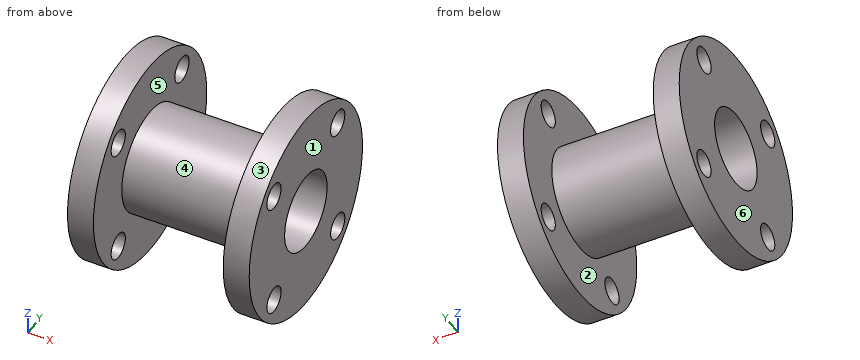
from build123d import *

# Parameters (mm, degrees)
F0_R     = 50.8
F0_R_2   = 6.35
F0_R_3   = 25.4
F1_DEPTH = 12.7
F0_R_4   = 19.05
F2_DEPTH = 88.9
F3_R     = 50.8
F3_R_2   = 6.35
F3_R_3   = 25.4
F4_DEPTH = 12.7


with BuildPart() as f1:
    # F0 (on Right) → F1 (new body)
    with BuildSketch(Plane.YZ):
        Circle(F0_R)
        with Locations((-28.575, -28.575)):
            Circle(F0_R_2, mode=Mode.SUBTRACT)
        Circle(F0_R_3, mode=Mode.SUBTRACT)
        with Locations((28.575, -28.575)):
            Circle(F0_R_2, mode=Mode.SUBTRACT)
        with Locations((-28.575, 28.575)):
            Circle(F0_R_2, mode=Mode.SUBTRACT)
        with Locations((28.575, 28.575)):
            Circle(F0_R_2, mode=Mode.SUBTRACT)
    extrude(amount=F1_DEPTH)

    # F0 (on Right) → F2 (join)
    with BuildSketch(Plane.YZ):
        Circle(F0_R_3)
        Circle(F0_R_4, mode=Mode.SUBTRACT)
    extrude(amount=F2_DEPTH)

    # F3 (on face) → F4 (join)
    with BuildSketch(Plane.YZ.offset(88.9)):
        Circle(F3_R)
        with Locations((-28.575, -28.575)):
            Circle(F3_R_2, mode=Mode.SUBTRACT)
        Circle(F3_R_3, mode=Mode.SUBTRACT)
        with Locations((28.575, -28.575)):
            Circle(F3_R_2, mode=Mode.SUBTRACT)
        with Locations((-28.575, 28.575)):
            Circle(F3_R_2, mode=Mode.SUBTRACT)
        with Locations((28.575, 28.575)):
            Circle(F3_R_2, mode=Mode.SUBTRACT)
    extrude(amount=-F4_DEPTH)


solid = f1.part
For this review, take the finished solid that the model builds, in its own axes (mm). Face numbers are marked on the shaded views. A direction names the side the tool comes from. Round coordinates to 2 decimals unless told otherwise and drop trailing zeros. Write each loop counter-clockwise with the first axis right and the second up, starting at its lowest first coordinate (ties: lowest second). Pieces come first, ordered by that corner, then holes. Notation, with made-up numbers: (-35.5, 69) -> (-24.5, 69) arc R26 ccw to (-24.5, 97) -> close; hole circle Ø10 at (-32, 41). An arc over 180 degrees is marked (long way). Use CSV: the item, a comma, the result in double quotes.
(1) Consider section D-D, the plane x = 36. Give the boundary of the cut face in (y, z).
Computed values:
outline,"circle Ø50.8 at (0, 0); hole circle Ø38.1 at (0, 0)"
(2) Clearance check with flat-ended pins moving along their axes: P1, Ø2, axis at x = 72, z = 8.5, coming from the -Y side; P2, Ø4, axis at x = 78, z = -26.5, coming from the +Y side; P3, Ø1.5, axis at x = 59, z = -3, coming from the -Y side. State where each tip first meets the part, or that it passes through.
Computed values:
P1,"y = -24.27"
P2,"y = 44.5"
P3,"y = -25.3"
(3) Consider section A-A, the plane z = 0. Give the boundary of the cut face in (x, y).
Computed values:
outline,"(0, -50.8) -> (12.7, -50.8) -> (12.7, -25.4) -> (76.2, -25.4) -> (76.2, -50.8) -> (88.9, -50.8) -> (88.9, -19.05) -> (0, -19.05) -> close; (0, 19.05) -> (88.9, 19.05) -> (88.9, 50.8) -> (76.2, 50.8) -> (76.2, 25.4) -> (12.7, 25.4) -> (12.7, 50.8) -> (0, 50.8) -> close"
(4) To check wall thickness, follow L1, parallel to X at y = -31, z = -6; L2, parallel to Z at x = 81.5, y = -29.5; L3, parallel to Z at x = 36, y = 0. State the ranges of each line that lie inside material, in increasing order. Write a range as [from, to].
Computed values:
L1,"[0, 12.7], [76.2, 88.9]"
L2,"[-41.36, -34.86], [-22.29, 22.29], [34.86, 41.36]"
L3,"[-25.4, -19.05], [19.05, 25.4]"
(5) Consider section C-C, the plane y = -31. Give the boundary of the cut face in (x, z).
Computed values:
outline,"(0, -40.24) -> (12.7, -40.24) -> (12.7, -34.44) -> (0, -34.44) -> close; (0, -22.71) -> (12.7, -22.71) -> (12.7, 22.71) -> (0, 22.71) -> close; (0, 34.44) -> (12.7, 34.44) -> (12.7, 40.24) -> (0, 40.24) -> close; (76.2, -40.24) -> (88.9, -40.24) -> (88.9, -34.44) -> (76.2, -34.44) -> close; (76.2, -22.71) -> (88.9, -22.71) -> (88.9, 22.71) -> (76.2, 22.71) -> close; (76.2, 34.44) -> (88.9, 34.44) -> (88.9, 40.24) -> (76.2, 40.24) -> close"
(6) For the marked faces 5 and 6, list the 3-axis set-ups (+Z, -Z, +X, -X, +Y, -Y) from which the entire face can be reached by the end or side of a thin tool; tool diameter is ignored.
Computed values:
face 5,"none"
face 6,"+Z, -Z, -X, +Y, -Y"
(7) Draft analysis for pull direction X (two halves, no side actions). For the marked faces 1, 2, 3 and 4, state which applies: +X half, -X half, draft (parallel to the pull), parting line (faces both ways), or undercut.
Computed values:
face 1,"+X half"
face 2,"undercut"
face 3,"draft"
face 4,"undercut"
